Could you check a few things on this model? Use its own coordinates, in mm. Give positions to 0.01 mm unless a question says otherwise; leave off trailing zeros. Loops run counter-clockwise (first coordinate to the right, second up) from the corner with the lowest first, then second, coordinate; pieces in that order, holes last. Notation, with made-up numbers: (-16, 20.25) -> (28, 20.25) arc R27 ccw to (28, 37.25) -> close; hole circle Ø8 at (-40, 15.5). An arc over 180 degrees is marked (long way). Write each question's results on one line, items separated by ' | '. Start each with the question number.
Q1. If I drill on line 1 along Y through (x, z) = (-5, 92); line 2 along Y through (x, z) = (0, 116); line 3 along Y through (x, z) = (9, 13.5), over which ranges is the centre line in solid material (lowest first)?
Q2. Will this pin go through, and if not, where does the flat tip stop? P1, Ø3, axis at y = 0.5, z = 116, coming from the -X side.
Q3. If we section it at A-A, the plane y = 0: List the corners of the cut face in (x, z) for me, plus the area to 3 significant figures.
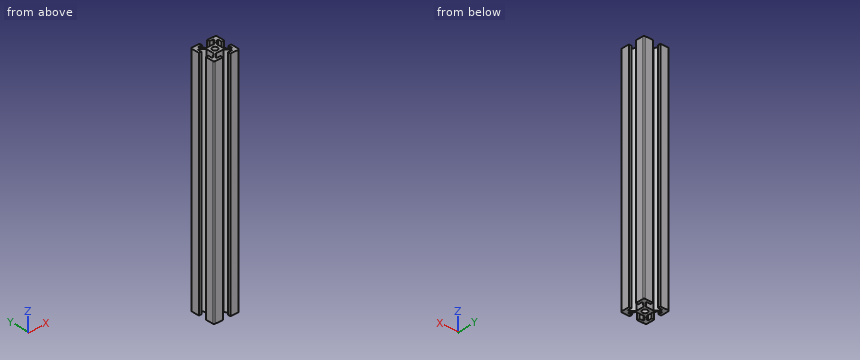
from build123d import *

# Parameters (mm, degrees)
SKETCH1_R           = 2.1
BOSS_EXTRUDE1_DEPTH = 180


with BuildPart() as part:
    # Sketch1 → Boss-Extrude1 (new body)
    with BuildSketch(Plane(origin=(0, 0, 0), x_dir=(-1, 0, 0), z_dir=(0, 0, -1))):
        with BuildLine():
            Line((6, -8), (3, -8))
            Line((3, -8), (3, -10))
            Line((3, -10), (9, -10))
            ThreePointArc((9, -10), (9.707106781, -9.707106781), (10, -9))
            Line((10, -9), (10, -3))
            Line((10, -3), (8, -3))
            Line((8, -3), (8, -6))
            Line((8, -6), (7, -6))
            Line((7, -6), (4, -3))
            Line((4, -3), (4, 3))
            Line((4, 3), (7, 6))
            Line((7, 6), (8, 6))
            Line((8, 6), (8, 3))
            Line((8, 3), (10, 3))
            Line((10, 3), (10, 9))
            ThreePointArc((10, 9), (9.707106781, 9.707106781), (9, 10))
            Line((9, 10), (3, 10))
            Line((3, 10), (3, 8))
            Line((3, 8), (6, 8))
            Line((6, 8), (6, 7))
            Line((6, 7), (3, 4))
            Line((3, 4), (-3, 4))
            Line((-3, 4), (-6, 7))
            Line((-6, 7), (-6, 8))
            Line((-6, 8), (-3, 8))
            Line((-3, 8), (-3, 10))
            Line((-3, 10), (-9, 10))
            ThreePointArc((-9, 10), (-9.707106781, 9.707106781), (-10, 9))
            Line((-10, 9), (-10, 3))
            Line((-10, 3), (-8, 3))
            Line((-8, 3), (-8, 6))
            Line((-8, 6), (-7, 6))
            Line((-7, 6), (-4, 3))
            Line((-4, 3), (-4, -3))
            Line((-4, -3), (-7, -6))
            Line((-7, -6), (-8, -6))
            Line((-8, -6), (-8, -3))
            Line((-8, -3), (-10, -3))
            Line((-10, -3), (-10, -9))
            ThreePointArc((-10, -9), (-9.707106781, -9.707106781), (-9, -10))
            Line((-9, -10), (-3, -10))
            Line((-3, -10), (-3, -8))
            Line((-3, -8), (-6, -8))
            Line((-6, -8), (-6, -7))
            Line((-6, -7), (-3, -4))
            Line((-3, -4), (3, -4))
            Line((3, -4), (6, -7))
            Line((6, -7), (6, -8))
        make_face()
        Circle(SKETCH1_R, mode=Mode.SUBTRACT)
    extrude(amount=-BOSS_EXTRUDE1_DEPTH)


solid = part.part
Final values:
1) line 1: y = -10 to -8, -6 to -4, 4 to 6, 8 to 10 | line 2: y = -4 to -2.1, 2.1 to 4 | line 3: y = -10 to -3, 3 to 10
2) P1: stops at x = -4
3) outline: (-4, 0) -> (-2.1, 0) -> (-2.1, 180) -> (-4, 180) -> close; (2.1, 0) -> (4, 0) -> (4, 180) -> (2.1, 180) -> close | area: 684 mm²
